The listing builds one solid part. Answer for the finished solid, in the listing's coordinates (mm). A direction names the side the tool comes from. Coordinates: 2 decimals unless noted, no trailing zeros. Write each loop counter-clockwise with the first axis right and the second up, starting at its lowest first coordinate (ties: lowest second). Pieces come first, ordered by that corner, then holes.
from build123d import *

# Parameters (mm, degrees)
ESQUISSE1_R             = 47.9
BOSS_EXTRU_1_DEPTH      = 10
ESQUISSE2_R             = 60
BOSS_EXTRU_2_DEPTH      = 10
ENL_V_START             = -10
ESQUISSE4_R             = 47.9
ESQUISSE4_R_2           = 46.5
ENL_V_MAT_EXTRU_1_DEPTH = 10
ESQUISSE5_R             = 5
ENL_V_MAT_EXTRU_2_DEPTH = 88.177978871


with BuildPart() as part:
    # Esquisse1 → Boss.-Extru.1 (new body)
    with BuildSketch(Plane(origin=(0, 0, 0), x_dir=(1, 0, 0), z_dir=(0, 1, 0))):
        with Locations(Location((0, 0, 0), (0, 0, 270))):
            Circle(ESQUISSE1_R)
    extrude(amount=BOSS_EXTRU_1_DEPTH)

    # Esquisse2 → Boss.-Extru.2 (add)
    with BuildSketch(Plane.XZ):
        with Locations(Location((0, 0, 0), (0, 0, 270))):
            Circle(ESQUISSE2_R)
    extrude(amount=BOSS_EXTRU_2_DEPTH)

    # Esquisse4 → Enlèv. mat.-Extru.1 (cut)
    with BuildSketch(Plane(origin=(0, 10, 0), x_dir=(1, 0, 0), z_dir=(0, 1, 0)).offset(ENL_V_START)):
        Circle(ESQUISSE4_R)
        with Locations(Location((0, 0, 0), (0, 0, 270))):
            Circle(ESQUISSE4_R_2, mode=Mode.SUBTRACT)
    extrude(amount=ENL_V_MAT_EXTRU_1_DEPTH, mode=Mode.SUBTRACT)

    # Esquisse5 → Enlèv. mat.-Extru.2 (cut, through all)
    with BuildSketch(Plane(origin=(0, 10, 0), x_dir=(1, 0, 0), z_dir=(0, 1, 0))):
        with Locations(Location((0, 0, 0), (0, 0, 270))):
            Circle(ESQUISSE5_R)
    extrude(amount=-ENL_V_MAT_EXTRU_2_DEPTH, mode=Mode.SUBTRACT)


solid = part.part
Q1. Determine the mould class of faces 3 (the face through (46.1, 4.9, -6.1)), 4 (the face through (-4.88, 0.14, -1.08)), 5 (the face through (1, -10, -12)) for opening direction X: released by +X, released by -X, zero draft, split by the parting line, or undercut.
Answers below:
face 3: split by the parting line
face 4: undercut
face 5: zero draft
Q2. Given pin 1 (8 mm diameter, centred on x = -9, y = 7.5, fed in from +Z); pin 2 (12 mm diameter, centred on y = -5, z = 6.5, fed in from +X); pin 3 (3 mm diameter, centred on x = 30.5, y = 7, fed in from +Z); pin 4 (13 mm diameter, centred on x = 0, z = 0, fed in from -Y), each flat-ended and moving along its own axis, determine where each tip first touches the part or whether it passes through.
Answers below:
pin 1: stops at z = 46.23
pin 2: stops at x = 60
pin 3: stops at z = 36.35
pin 4: stops at y = -10
Q3. Find the intervals of material crossed by probe 1 along X at (y, z) = (-2, 0); probe 2 along X at (y, z) = (5.25, 0); probe 3 along Y at (x, z) = (53.5, 3), in increasing order.
Answers below:
probe 1: x = -60 to -5, 5 to 60
probe 2: x = -46.5 to -5, 5 to 46.5
probe 3: y = -10 to 0
Q4. The part is cut by section B-B, the plane x = 0. Write down the section's boundary in (y, z).
Answers below:
outline: (-10, -60) - (0, -60) - (0, -46.5) - (10, -46.5) - (10, -5) - (-10, -5) - close; (-10, 5) - (10, 5) - (10, 46.5) - (0, 46.5) - (0, 60) - (-10, 60) - close
Q5. The part is cut by section D-D, the plane x = -19. Write down the section's boundary in (y, z), then the cut area to 3 significant figures.
Answers below:
outline: (-10, -56.91) - (0, -56.91) - (0, -42.44) - (10, -42.44) - (10, 42.44) - (0, 42.44) - (0, 56.91) - (-10, 56.91) - close
area: 1,990 mm2
Q6. The part is cut by section A-A, the plane z = 0. Write down the section's boundary in (x, y).
Answers below:
outline: (-60, -10) - (-5, -10) - (-5, 10) - (-46.5, 10) - (-46.5, 0) - (-60, 0) - close; (5, -10) - (60, -10) - (60, 0) - (46.5, 0) - (46.5, 10) - (5, 10) - close
Q7. The part is cut by section C-C, the plane y = -4.5. Write down the section's boundary in (x, z), then the cut area to 3 significant figures.
Answers below:
outline: circle Ø120 at (0, 0); hole circle Ø10 at (0, 0)
area: 11,200 mm2
Q8. Which of the six approach directions +Z, -Z, +X, -X, +Y, -Y give full straight-line access (tool end or side, diameter ignored) to faces 1 (the face through (2.64, -4.93, 59.94)), 2 (the face through (-35, 0, -31))?
Answers below:
face 1: +Y, -Y
face 2: +Y
